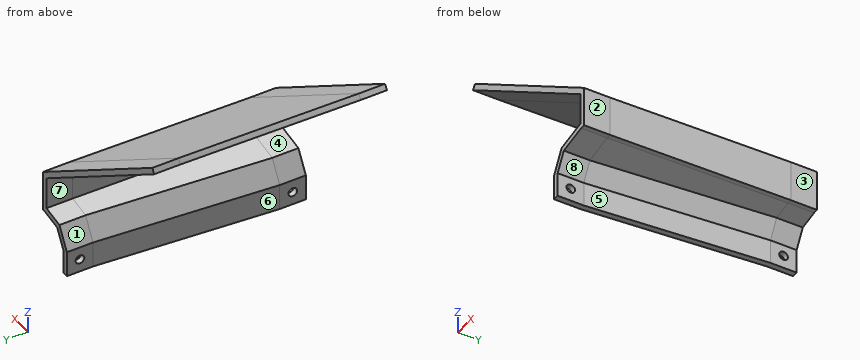
```python
from build123d import *

# Parameters (mm, degrees)
F3_W           = 18
F3_H           = 18
F3_R           = 3
F4_DEPTH       = 2
F5_W           = 18
F5_H           = 18
F5_R           = 3
F6_DEPTH       = 2
F8_DEPTH       = 9
F8_DEPTH_BACK  = 9
F10_DEPTH      = 9
F10_DEPTH_BACK = 9
F12_DEPTH      = 18
F14_DEPTH      = 18


with BuildPart() as f4:
    # F3 (on Right) → F4 (new body, symmetric)
    with BuildSketch(Plane.YZ):
        with Locations((70.25, 0)):
            Rectangle(F3_W, F3_H)
        with Locations((70.25, 0)):
            Circle(F3_R, mode=Mode.SUBTRACT)
    extrude(amount=F4_DEPTH, both=True)

    # F7 (on offset) → F8 (join, two sides)
    with BuildSketch(Plane.XZ.offset(-70.25)) as f8_sk:
        Polygon((6.5, 23.7224318643), (-2, 9), (2, 9), (2, 7.9282032303), (9.0314862988, 20.1070947526), (21.9667090059, 22.3879235173), (21.2721162952, 26.3271545293), align=None)
    extrude(amount=-F8_DEPTH)
    extrude(f8_sk.sketch, amount=F8_DEPTH_BACK)

    # F11 (on face) → F12 (join, through all)
    with BuildSketch(Plane(origin=(0, 79.25, 0), x_dir=(-1, 0, 0), z_dir=(0, 1, 0))):
        Polygon((-21.9667090059, 22.3879235173), (-21.2721162952, 26.3271545293), (-21.2721162952, 48.8271545293), (101.6006903482, 134.863619982), (99.7962957674, 138.4832676497), (-25.2721162952, 50.9094227315), (-25.2721162952, 22.3879235173), align=None)
    extrude(amount=-F12_DEPTH)



with BuildPart() as f6:
    # F5 (on offset) → F6 (new body, symmetric)
    with BuildSketch(Plane.YZ.offset(-10)):
        with Locations((-70.25, 0)):
            Rectangle(F5_W, F5_H)
        with Locations((-70.25, 0)):
            Circle(F5_R, mode=Mode.SUBTRACT)
    extrude(amount=F6_DEPTH, both=True)

    # F9 (on offset) → F10 (join, two sides)
    with BuildSketch(Plane.XZ.offset(70.25)) as f10_sk:
        Polygon((18.1657705663, 27.542691773), (-3.5, 23.7224318643), (-12, 9), (-8, 9), (-8, 7.9282032303), (-0.9685137012, 20.1070947526), (18.8603632769, 23.603460761), align=None)
    extrude(amount=F10_DEPTH)
    extrude(f10_sk.sketch, amount=-F10_DEPTH_BACK)

    # F13 (on face) → F14 (join, through all)
    with BuildSketch(Plane.XZ.offset(79.25)):
        Polygon((18.1657705663, 49.542691773), (18.1657705663, 27.542691773), (18.8603632769, 23.603460761), (22.1657705663, 23.603460761), (22.1657705663, 51.6249599752), (-102.4127303317, 138.8557654028), (-104.7070360771, 135.5791572257), align=None)
    extrude(amount=-F14_DEPTH)


with BuildPart() as f4_1:
    add(f4.part)

    add(f6.part)  # F15 merges F6
    # F12_face (on face) → F15 section 0
    with BuildSketch(Plane(origin=(-21.9904596416, 61.25, 69.4287440583), x_dir=(1, 0, 0), z_dir=(0, -1, 0))):
        Polygon((19.9904596416, -60.4287440583), (19.9904596416, -78.4287440583), (23.9904596416, -78.4287440583), (23.9904596416, -61.500540828), (31.0219459404, -49.3216493057), (43.9571686475, -47.040820541), (47.2625759368, -47.040820541), (47.2625759368, -18.5193213268), (-77.8058361258, 69.0545235914), (-79.6102307066, 65.4348759237), (43.2625759368, -20.601589529), (43.2625759368, -43.101589529), (28.4904596416, -45.706312194), align=None)
    # F14_face (on face) → F15 section 1
    with BuildSketch(Plane(origin=(-25.2803198576, -61.25, 68.6471085342), x_dir=(-1, 0, 0), z_dir=(0, 1, 0))):
        Polygon((-13.2803198576, -77.6471085342), (-13.2803198576, -59.6471085342), (-21.7803198576, -44.9246766699), (-43.4460904239, -41.1044167612), (-43.4460904239, -19.1044167612), (79.4267162195, 66.9320486914), (77.1324104741, 70.2086568686), (-47.4460904239, -17.022148559), (-47.4460904239, -45.0436477733), (-44.1406831345, -45.0436477733), (-24.3118061564, -48.5400137817), (-17.2803198576, -60.7189053039), (-17.2803198576, -77.6471085342), align=None)
    loft()


solid = f4_1.part
```
Input: part model. Units: mm. Frame: model coordinates. Face numbers are marked on the shaded views. A direction names the side the tool comes from. Coordinates: 2 decimals unless noted, no trailing zeros. Order: outer loops, then holes, each group sorted by start corner. A loop starts at its lowest first (then second) coordinate and runs counter-clockwise, first axis right, second up. Notation, with made-up numbers: (53.5, 21.5) - (103.5, 21.5) arc R8 ccw to (103.5, 29.5) - close; hole circle Ø11 at (3, 59). An arc over 180 degrees is marked (long way). Put each result on its own line as item: value.
1. Line query: line 1 along Z through (x, y) = (-10.7, -70.25); line 2 along Z through (x, y) = (0, 70); line 3 along X through (y, z) = (-70, 114). Output: solid intervals per line, ascending.
Report:
line 1: z = -9 to -3, 3 to 11.25, 69.75 to 74.64
line 2: z = -9 to -2.99, 2.99 to 12.46, 63.72 to 68.61
line 3: x = -73.89 to -66.92
2. Cut plane B-B on z = 0. Return the cut outline in (x, y).
Report:
outline: (-12, -79.25) - (-8, -79.25) - (-8, -73.25) - (-12, -73.25) - close; (-12, -67.25) - (-8, -67.25) - (-8, -61.25) - (2, 61.25) - (2, 67.25) - (-2, 67.25) - (-2, 61.25) - (-12, -61.25) - close; (-2, 73.25) - (2, 73.25) - (2, 79.25) - (-2, 79.25) - close
3. Cut plane C-C on y = -70.25. Return the cut outline in (x, z), then the cut area to 3 significant figures.
Report:
outline: (-104.71, 135.58) - (18.17, 49.54) - (18.17, 27.54) - (-3.5, 23.72) - (-12, 9) - (-12, 3) - (-8, 3) - (-8, 7.93) - (-0.97, 20.11) - (18.86, 23.6) - (22.17, 23.6) - (22.17, 51.62) - (-102.41, 138.86) - close; (-12, -9) - (-8, -9) - (-8, -3) - (-12, -3) - close
area: 903 mm2
4. Draft query along Z for the marked faces 6, 7 and 8. Return one class per face: pulls with the +Z half, pulls with the -Z half, needs draft (parallel to the pull), parting line crosses it, or undercut.
Report:
face 6: needs draft
face 7: undercut
face 8: pulls with the -Z half
5. Contact query for flat-ended pins moving along their axis: pin 1 Ø13.5 at (y, z) = (69.5, -3.5) entering from +X; pin 2 Ø5.5 at (y, z) = (-72, 31) entering from +X; pin 3 Ø3.5 at (x, y) = (21, -66) entering from -Z. Output: stop coordinate, or through.
Report:
pin 1: stops at x = 2
pin 2: stops at x = 22.17
pin 3: stops at z = 23.6
6. Cut plane A-A on y = 70.25. Return the cut outline in (x, z), then the cut area to 3 significant figures.
Report:
outline: (-101.6, 134.86) - (21.27, 48.83) - (21.27, 26.33) - (6.5, 23.72) - (-2, 9) - (-2, 3) - (2, 3) - (2, 7.93) - (9.03, 20.11) - (21.97, 22.39) - (25.27, 22.39) - (25.27, 50.91) - (-99.8, 138.48) - close; (-2, -9) - (2, -9) - (2, -3) - (-2, -3) - close
area: 878 mm2
7. Reachability of the marked faces 1, 2, 3, 4 and 5 from +Z, -Z, +X, -X, +Y, -Y: full face, straight path, thin tool, end or side. Return the list, or none.
Report:
face 1: -X, +Y
face 2: +Z, -Z, +X, -Y
face 3: +Z, -Z, +X, +Y, -Y
face 4: -X, +Y, -Y
face 5: -Z, +X, -Y
